Drawing for the job (mm, zero at the part's lowest x, y, z). A direction names the side the tool comes from. Give positions to 0.01 mm unless a question says otherwise; leave off trailing zeros. Loops run counter-clockwise (first coordinate to the right, second up) from the corner with the lowest first, then second, coordinate; pieces in that order, holes last. Notation, with made-up numbers: (-2, 1) -> (51, 1) arc R11 cw to (51, 19) -> close; hole circle Ø5 at (-1.75, 22). An arc over 180 degrees is marked (long way). Answer in a Markdown table with one row per item. Add a question column.
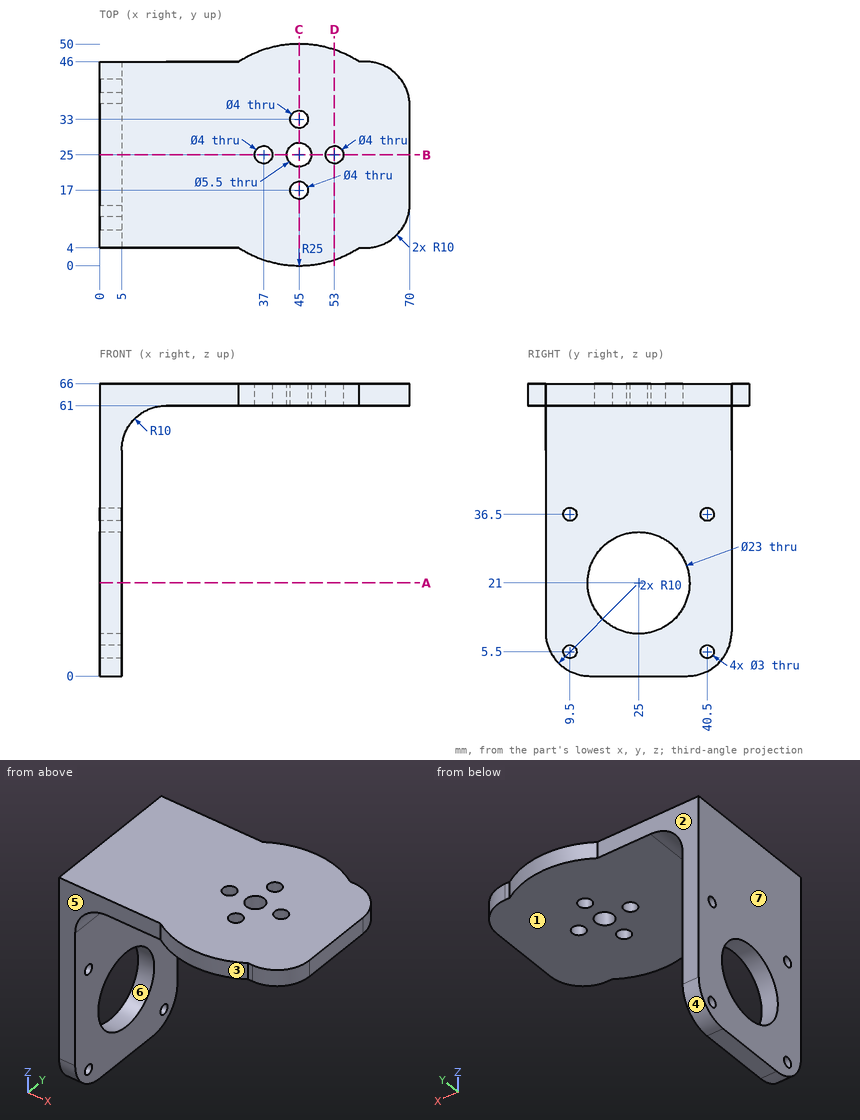
(1) Two-plate mould, pull along Y, no slides. Class the marked faces 4, 5, 6 and 7: released by +Y, released by -Y, zero draft, split by the parting line, or undercut.
(2) Saw through at C-C, the plane x = 45. List the corners of the cut face in (y, z), then the cut area to 4 significant figures.
(3) Saw through at B-B, the plane y = 25. List the corners of the cut face in (x, z).
(4) Saw through at D-D, the plane x = 53. List the corners of the cut face in (y, z).
(5) Saw through at A-A, the plane z = 21. List the corners of the cut face in (x, y).
(6) Flat gauge pins, fed straight in: pin 1 Ø10 at (y, z) = (39.5, 38.5) entering from -X; pin 2 Ø25 at (x, z) = (9, 34) entering from +Y; pin 3 Ø21 at (y, z) = (24, 32.5) entering from +X; pin 4 Ø1.6 at (x, z) = (59, 63.5) entering from -Y. Where does each tip first touch, or does it go through?
(7) Wall check: line 1 along Y through (x, z) = (45, 64.5); line 2 along Y through (x, z) = (2.3, 36.5); line 3 along Y through (x, z) = (3, 5). Give the ranges that are in metal, low to high. Write a range as from..to.
(8) 3-axis set-ups, long thin cutter, end or side, ignore diameter. For the marked faces 1, 2 and 3: which of +Z, -Z, +X, -X, +Y, -Y reach the whole face in a straight line?
Worked answers:
| question | item | result |
|---|---|---|
| 1 | face 4 | released by +Y |
| 1 | face 5 | released by -Y |
| 1 | face 6 | undercut |
| 1 | face 7 | zero draft |
| 2 | outline | (0, 61) -> (15, 61) -> (15, 66) -> (0, 66) -> close; (19, 61) -> (22.25, 61) -> (22.25, 66) -> (19, 66) -> close; (27.75, 61) -> (31, 61) -> (31, 66) -> (27.75, 66) -> close; (35, 61) -> (50, 61) -> (50, 66) -> (35, 66) -> close |
| 2 | area | 182.5 mm^2 |
| 3 | outline | (0, 0) -> (5, 0) -> (5, 9.5) -> (0, 9.5) -> close; (0, 32.5) -> (5, 32.5) -> (5, 51) arc R10 cw to (15, 61) -> (35, 61) -> (35, 66) -> (0, 66) -> close; (39, 61) -> (42.25, 61) -> (42.25, 66) -> (39, 66) -> close; (47.75, 61) -> (51, 61) -> (51, 66) -> (47.75, 66) -> close; (55, 61) -> (70, 61) -> (70, 66) -> (55, 66) -> close |
| 4 | outline | (1.31, 61) -> (23, 61) -> (23, 66) -> (1.31, 66) -> close; (27, 61) -> (48.69, 61) -> (48.69, 66) -> (27, 66) -> close |
| 5 | outline | (0, 4) -> (5, 4) -> (5, 13.5) -> (0, 13.5) -> close; (0, 36.5) -> (5, 36.5) -> (5, 46) -> (0, 46) -> close |
| 6 | pin 1 | x = 0 |
| 6 | pin 2 | y = 46 |
| 6 | pin 3 | x = 5 |
| 6 | pin 4 | y = 3.77 |
| 7 | line 1 | 0..15, 19..22.25, 27.75..31, 35..50 |
| 7 | line 2 | 4..8, 11..39, 42..46 |
| 7 | line 3 | 5.34..8.09, 10.91..39.09, 41.91..44.66 |
| 8 | face 1 | -Z, +X, +Y, -Y |
| 8 | face 2 | +Z, -Z, -X, +Y |
| 8 | face 3 | +Z, -Z, -Y |
